Autodesk Inventor part; units mm, degrees
ref_plane "YZ Plane" through (0, 0, 0) normal (1, 0, 0) x (0, 1, 0)
ref_plane "XZ Plane" through (0, 0, 0) normal (0, 1, 0) x (-1, 0, 0)
ref_plane "XY Plane" through (0, 0, 0) normal (0, 0, 1) x (1, 0, 0)
sketch "Sketch1" plane through (0, 0, 0) normal (0, 0, 1) x (1, 0, 0)
  line L0 (-43.5457, 39.1136) -> (-3.5457, 39.1136)
  line L1 (-3.5457, 39.1136) -> (-3.5457, -4.8864)
  line L2 (-3.5457, -4.8864) -> (-43.5457, -4.8864)
  line L3 (-43.5457, -4.8864) -> (-43.5457, 39.1136)
  point P0 (0, 0)
  dimension "d0" = 40
  dimension "d1" = 44
extrude "Extrusion1" add sketch "Sketch1" along normal blind 1.2
sketch "Sketch2" plane through (0, 0, 1.2) normal (0, 0, 1) x (1, 0, 0)
  line L0 (-45.5457, 41.1136) -> (-1.5457, 41.1136)
  line L1 (-1.5457, 41.1136) -> (-1.5457, -6.8864)
  line L2 (-1.5457, -6.8864) -> (-45.5457, -6.8864)
  line L3 (-45.5457, -6.8864) -> (-45.5457, 41.1136)
  line L4 (-3.5457, 39.1136) -> (-43.5457, 39.1136)
  line L5 (-43.5457, -4.8864) -> (-3.5457, -4.8864)
  line L6 (-3.5457, -4.8864) -> (-3.5457, 39.1136)
  line L7 (-43.5457, 39.1136) -> (-43.5457, -4.8864)
  point P0 (0, 0)
  dimension "d4" = 2
  dimension "d5" = 2
  dimension "d6" = 2
  dimension "d7" = 2
extrude "Extrusion2" add sketch "Sketch2" along normal blind 1.2 contours L0 L1 L2 L3 | L6 L5 L7 L4
sketch "Sketch3" plane through (0, 0, 2.4) normal (0, 0, 1) x (1, 0, 0)
  line L0 (-33.5457, 20.1136) -> (-13.5457, 20.1136)
  line L1 (-13.5457, 20.1136) -> (-13.5457, 7.1136)
  line L2 (-13.5457, 7.1136) -> (-33.5457, 7.1136)
  line L3 (-33.5457, 7.1136) -> (-33.5457, 20.1136)
  line L4 (-43.5457, -4.8864) -> (-3.5457, -4.8864)
  line L5 (-45.5457, 41.1136) -> (-45.5457, -6.8864)
  line L6 (-1.5457, -6.8864) -> (-1.5457, 41.1136)
  point P0 (0, 0)
  dimension "d10" = 12
  dimension "d11" = 25
  dimension "d12" = 12
  dimension "d13" = 12
extrude "Extrusion3" cut sketch "Sketch3" against normal blind 3
properties part number "Front"
The listing builds one solid part. Answer for the finished solid, in the listing's coordinates (mm). A direction names the side the tool comes from. Give positions to 0.01 mm unless a question says otherwise; leave off trailing zeros. Loops run counter-clockwise (first coordinate to the right, second up) from the corner with the lowest first, then second, coordinate; pieces in that order, holes last. Notation, with made-up numbers: (81, 28) - (130, 28) arc R14 cw to (130, 52) - close; hole circle Ø7 at (50.5, 59.25). An arc over 180 degrees is marked (long way). Use one line per item in the form item = value.
1. Given pin 1 Ø0.6 at (y, z) = (10.5, 0.5) entering from +X; pin 2 Ø1 at (x, z) = (-33, 0.5) entering from -Y; pin 3 Ø0.6 at (x, z) = (-28, 0.5) entering from +Y, each flat-ended and moving along its own axis, determine where each tip first touches the part or whether it passes through.
Calculated:
pin_1 = -3.55
pin_2 = -4.89
pin_3 = 39.11
2. Find the intervals of material crossed by line 1 along Y through (x, z) = (-14, 1.05); line 2 along X through (y, z) = (14.5, 0.65); line 3 along X through (y, z) = (19, 1.6), in increasing order. Write a range as [from, to].
Calculated:
line_1 = [-4.89, 7.11], [20.11, 39.11]
line_2 = [-43.55, -33.55], [-13.55, -3.55]
line_3 = [-45.55, -33.55], [-13.55, -1.55]
3. Section C-C on y = 13.5 is taken. Give the vertices of the cut face in (x, z), then the cut area to 3 significant figures.
Calculated:
outline = (-45.55, 1.2) - (-43.55, 1.2) - (-43.55, 0) - (-33.55, 0) - (-33.55, 2.4) - (-45.55, 2.4) - close; (-13.55, 0) - (-3.55, 0) - (-3.55, 1.2) - (-1.55, 1.2) - (-1.55, 2.4) - (-13.55, 2.4) - close
area = 52.8 mm^2
4. Section D-D on x = -43 is taken. Give the vertices of the cut face in (y, z).
Calculated:
outline = (-6.89, 1.2) - (-4.89, 1.2) - (-4.89, 0) - (39.11, 0) - (39.11, 1.2) - (41.11, 1.2) - (41.11, 2.4) - (-6.89, 2.4) - close
5. Section A-A on z = 1.75 is taken. Give the vertices of the cut face in (x, y), then the cut area to 3 significant figures.
Calculated:
outline = (-45.55, -6.89) - (-1.55, -6.89) - (-1.55, 41.11) - (-45.55, 41.11) - close; hole (-33.55, 7.11) - (-13.55, 7.11) - (-13.55, 20.11) - (-33.55, 20.11) - close
area = 1,850 mm^2
6. The mould has two halves that part along Y. Classify faces 4 (the face through (-13.546, 14, 1)), 5 (the face through (-23, -6.886, 2)), 6 (the face through (-45.546, 17, 2)): pulls with the +Y half, pulls with the -Y half, needs draft (parallel to the pull), parting line crosses it, or undercut.
Calculated:
face_4 = undercut
face_5 = pulls with the -Y half
face_6 = needs draft
7. Section B-B on x = -25.5 is taken. Give the vertices of the cut face in (y, z).
Calculated:
outline = (-6.89, 1.2) - (-4.89, 1.2) - (-4.89, 0) - (7.11, 0) - (7.11, 2.4) - (-6.89, 2.4) - close; (20.11, 0) - (39.11, 0) - (39.11, 1.2) - (41.11, 1.2) - (41.11, 2.4) - (20.11, 2.4) - close
8. Which of the six approach directions +Z, -Z, +X, -X, +Y, -Y give full straight-line access (tool end or side, diameter ignored) to faces 1 (the face through (-3.546, 17, 1)), 2 (the face through (-23, -4.886, 1)), 3 (the face through (-33.546, 14, 1))?
Calculated:
face_1 = -Z, +X, +Y, -Y
face_2 = -Z, +X, -X, -Y
face_3 = +Z, -Z
